Autodesk Inventor part; units mm, degrees
ref_plane "YZ Plane" through (0, 0, 0) normal (1, 0, 0) x (0, 1, 0)
ref_plane "XZ Plane" through (0, 0, 0) normal (0, 1, 0) x (-1, 0, 0)
ref_plane "XY Plane" through (0, 0, 0) normal (0, 0, 1) x (1, 0, 0)
sketch "Sketch1" plane through (0, 0, 0) normal (0, 0, 1) x (1, 0, 0)
  circle A0 centre (0, 0) radius 1.25
  line L0 (0, 0) -> (16, 0) construction
  circle A1 centre (16, 0) radius 1.25
  arc A2 (0.367, 2.4729) -> (0.367, -2.4729) centre (0, 0) ccw
  arc A3 (15.633, -2.4729) -> (15.633, 2.4729) centre (16, 0) ccw
  arc A4 (0.367, 2.4729) -> (15.633, 2.4729) centre (8, 53.9096) ccw
  arc A5 (15.633, -2.4729) -> (0.367, -2.4729) centre (8, -53.9096) ccw
  dimension "d0" = 2.5
  dimension "d1" = 16
  dimension "d8" = 5
  dimension "d15" = 52
extrude "Extrusion1" add sketch "Sketch1" along normal blind 1.5
properties part number "linkageB"
Read the model definition and answer for the solid it produces. Units are mm, in the model's axes. Give positions to 0.01 mm unless a question says otherwise; leave off trailing zeros. Loops run counter-clockwise (first coordinate to the right, second up) from the corner with the lowest first, then second, coordinate; pieces in that order, holes last. Notation, with made-up numbers: (-15, 29) -> (3, 29) arc R20 cw to (3, 35) -> close; hole circle Ø2 at (-6.5, 3). An arc over 180 degrees is marked (long way). Use a Markdown table: item, result.
Q1. Determine the mould class of faces 1 (the face through (8.11, 1.91, 0.74)), 2 (the face through (8, 0, 0)) for opening direction X: pulls with the +X half, pulls with the -X half, needs draft (parallel to the pull), parting line crosses it, or undercut.
Solved:
| item | result |
|---|---|
| face 1 | undercut |
| face 2 | needs draft |
Q2. Section D-D, the plane y = 1 is taken. Determine the outline of the cut face in (x, z).
Solved:
| item | result |
|---|---|
| outline | (-2.29, 0) -> (-0.75, 0) -> (-0.75, 1.5) -> (-2.29, 1.5) -> close; (0.75, 0) -> (15.25, 0) -> (15.25, 1.5) -> (0.75, 1.5) -> close; (16.75, 0) -> (18.29, 0) -> (18.29, 1.5) -> (16.75, 1.5) -> close |
Q3. Section A-A, the plane x = 0 is taken. Determine the outline of the cut face in (y, z), then the cut area to 3 significant figures.
Solved:
| item | result |
|---|---|
| outline | (-2.5, 0) -> (-1.25, 0) -> (-1.25, 1.5) -> (-2.5, 1.5) -> close; (1.25, 0) -> (2.5, 0) -> (2.5, 1.5) -> (1.25, 1.5) -> close |
| area | 3.75 mm^2 |
Q4. Section B-B, the plane y = 0 is taken. Determine the outline of the cut face in (x, z).
Solved:
| item | result |
|---|---|
| outline | (-2.5, 0) -> (-1.25, 0) -> (-1.25, 1.5) -> (-2.5, 1.5) -> close; (1.25, 0) -> (14.75, 0) -> (14.75, 1.5) -> (1.25, 1.5) -> close; (17.25, 0) -> (18.5, 0) -> (18.5, 1.5) -> (17.25, 1.5) -> close |
Q5. Section C-C, the plane z = 0.9 is taken. Determine the outline of the cut face in (x, y), then the cut area to 3 significant figures.
Solved:
| item | result |
|---|---|
| outline | (0.37, -2.47) arc R52 cw to (15.63, -2.47) arc R2.5 ccw (long way) to (15.63, 2.47) arc R52 cw to (0.37, 2.47) arc R2.5 ccw (long way) to start; hole circle Ø2.5 at (0, 0); hole circle Ø2.5 at (16, 0) |
| area | 77.5 mm^2 |
Q6. Find the intervals of material crossed by line 1 along X through (y, z) = (0.8, 0.25); line 2 along X through (y, z) = (0.5, 1.1); line 3 along Y through (x, z) = (0, 1.25), in increasing order.
Solved:
| item | result |
|---|---|
| line 1 | x = -2.37 to -0.96, 0.96 to 15.04, 16.96 to 18.37 |
| line 2 | x = -2.45 to -1.15, 1.15 to 14.85, 17.15 to 18.45 |
| line 3 | y = -2.5 to -1.25, 1.25 to 2.5 |
